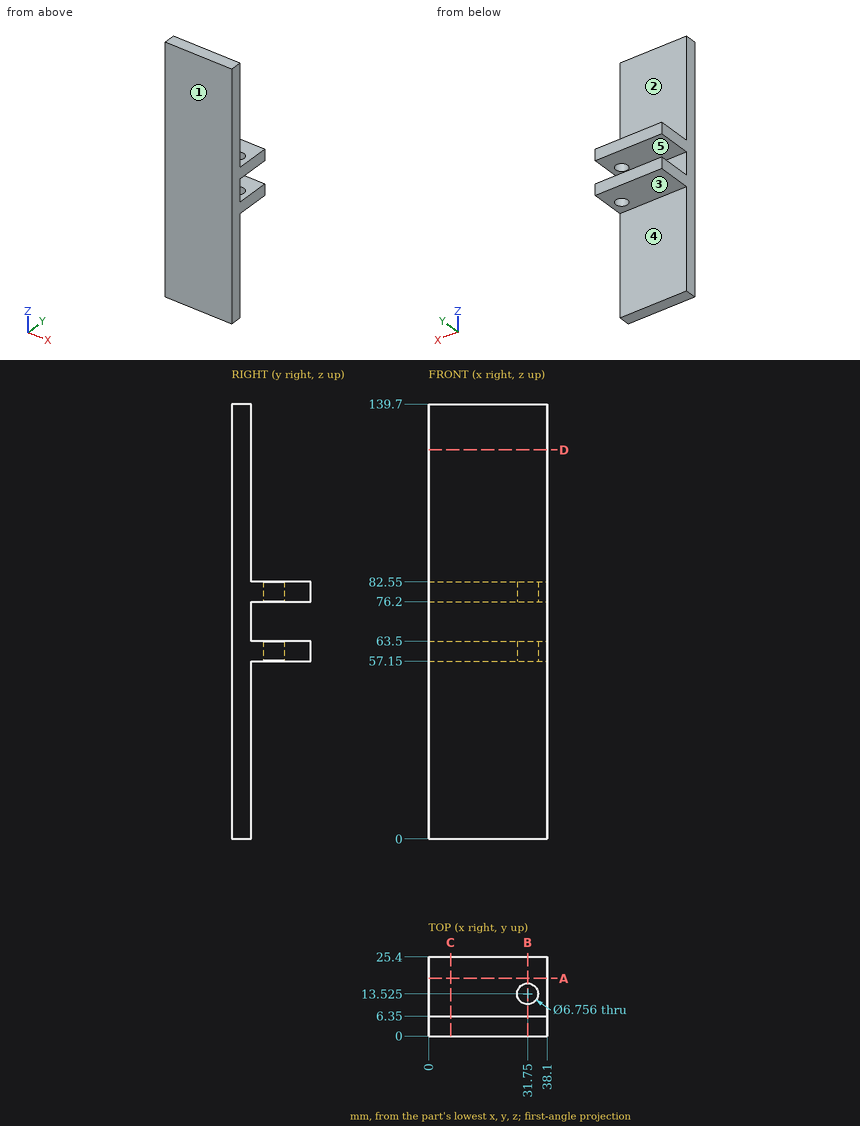
Part print with two shaded views. Sizes in mm from the minimum x, y, z corner. A direction names the side the tool comes from. Round coordinates to 2 decimals unless told otherwise and drop trailing zeros. Write each loop counter-clockwise with the first axis right and the second up, starting at its lowest first coordinate (ties: lowest second). Pieces come first, ordered by that corner, then holes. Notation, with made-up numbers: M -38.75,-6 L -20.75,-6 A19 ccw -20.75,19 Z; hole C 29.25,53 d6. An arc over 180 degrees is marked long. Put each result on its own line as item: value. Start each with the question number.
1) Pull direction Z, two halves, no side cores. Call the marked faces 3, 4 and 5: pulls with the +Z half, pulls with the -Z half, needs draft (parallel to the pull), parting line crosses it, or undercut.
2) Saw through at A-A, the plane y = 18.5. Write the cut outline in (x, z), and give its area (3 significant figures).
3) Drill centre lines: probe 1 along Z at (x, y) = (22.5, 10); probe 2 along Y at (x, z) = (31.75, 62.25). Where is each one in solid material? Low to high. Write a range as [from, to].
4) Saw through at D-D, the plane z = 125. Write the cut outline in (x, y).
5) Pin check, flat tips, straight feed: pin 1 Ø5.5 at (x, y) = (16.5, 20.5) entering from +Z; pin 2 Ø8 at (x, y) = (33.5, 15) entering from -Z; pin 3 Ø11.5 at (x, z) = (24.5, 43) entering from +Y; pin 4 Ø8 at (x, z) = (19.5, 110.5) entering from -Y. Stop position of each tip, or through.
6) Saw through at B-B, the plane x = 31.75. Write the cut outline in (y, z).
7) Saw through at C-C, the plane x = 7. Write the cut outline in (y, z), and give its area (3 significant figures).
8) 3-axis set-ups, long thin cutter, end or side, ignore diameter. For the marked faces 1 and 2: which of +Z, -Z, +X, -X, +Y, -Y reach the whole face in a straight line?
Resolved:
1. face 3: pulls with the -Z half
1. face 4: needs draft
1. face 5: undercut
2. outline: M 0,57.15 L 38.1,57.15 L 38.1,63.5 L 0,63.5 Z; M 0,76.2 L 38.1,76.2 L 38.1,82.55 L 0,82.55 Z
2. area: 484 mm²
3. probe 1: [57.15, 63.5], [76.2, 82.55]
3. probe 2: [0, 10.15], [16.9, 25.4]
4. outline: M 0,0 L 38.1,0 L 38.1,6.35 L 0,6.35 Z
5. pin 1: z = 82.55
5. pin 2: z = 57.15
5. pin 3: y = 6.35
5. pin 4: y = 0
6. outline: M 0,0 L 6.35,0 L 6.35,57.15 L 10.15,57.15 L 10.15,63.5 L 6.35,63.5 L 6.35,76.2 L 10.15,76.2 L 10.15,82.55 L 6.35,82.55 L 6.35,139.7 L 0,139.7 Z; M 16.9,57.15 L 25.4,57.15 L 25.4,63.5 L 16.9,63.5 Z; M 16.9,76.2 L 25.4,76.2 L 25.4,82.55 L 16.9,82.55 Z
7. outline: M 0,0 L 6.35,0 L 6.35,57.15 L 25.4,57.15 L 25.4,63.5 L 6.35,63.5 L 6.35,76.2 L 25.4,76.2 L 25.4,82.55 L 6.35,82.55 L 6.35,139.7 L 0,139.7 Z
7. area: 1,130 mm²
8. face 1: +Z, -Z, +X, -X, -Y
8. face 2: +Z, +X, -X, +Y
